```python
from build123d import *

# Parameters (mm, degrees)
BOSS_EXTRUDE1_DEPTH     = 200
SKETCH4_R               = 30
CUT_EXTRUDE1_DEPTH      = 60
SHELL1_T                = -20
BOSS_EXTRUDE2_DEPTH     = 200
SKETCH6_R               = 115
CUT_EXTRUDE3_DEPTH      = 50
CUT_EXTRUDE4_DEPTH      = 716.017482304
CUT_EXTRUDE4_DEPTH_BACK = 716.017482304
SKETCH7_R               = 30


with BuildPart() as part:
    # Sketch1 → Boss-Extrude1 (new body)
    with BuildSketch(Plane(origin=(0, 0, 0), x_dir=(1, 0, 0), z_dir=(0, 1, 0))):
        with BuildLine():
            Line((-220, 270), (220, 270))
            ThreePointArc((220, 270), (255.355339059, 255.355339059), (270, 220))
            Line((270, 220), (270, -220))
            ThreePointArc((270, -220), (255.355339059, -255.355339059), (220, -270))
            Line((220, -270), (-220, -270))
            ThreePointArc((-220, -270), (-255.355339059, -255.355339059), (-270, -220))
            Line((-270, -220), (-270, 220))
            ThreePointArc((-270, 220), (-255.355339059, 255.355339059), (-220, 270))
        make_face()
    extrude(amount=BOSS_EXTRUDE1_DEPTH)

    # Sketch4 → Cut-Extrude1 (cut)
    with BuildSketch(Plane(origin=(0, 200, 0), x_dir=(1, 0, 0), z_dir=(0, 1, 0))):
        with Locations(Location((0, 160, 0), (0, 0, 270))):
            Circle(SKETCH4_R)
        with Locations(Location((160, 0, 0), (0, 0, 270))):
            Circle(SKETCH4_R)
        with Locations(Location((0, -160, 0), (0, 0, 270))):
            Circle(SKETCH4_R)
        with Locations(Location((-160, 0, 0), (0, 0, 270))):
            Circle(SKETCH4_R)
    extrude(amount=-CUT_EXTRUDE1_DEPTH, mode=Mode.SUBTRACT)

    # Shell1
    shell1_openings = [part.faces().sort_by_distance(p)[0] for p in [
        (0, 0, 0),
    ]]
    offset(amount=SHELL1_T, openings=shell1_openings, kind=Kind.INTERSECTION)

    # Sketch5 → Boss-Extrude2 (add)
    with BuildSketch(Plane(origin=(0, 0, 0), x_dir=(1, 0, 0), z_dir=(0, 1, 0))):
        with BuildLine():
            Line((-255, 305), (255, 305))
            ThreePointArc((255, 305), (290.355339059, 290.355339059), (305, 255))
            Line((305, 255), (305, -255))
            ThreePointArc((305, -255), (290.355339059, -290.355339059), (255, -305))
            Line((255, -305), (-255, -305))
            ThreePointArc((-255, -305), (-290.355339059, -290.355339059), (-305, -255))
            Line((-305, -255), (-305, 255))
            ThreePointArc((-305, 255), (-290.355339059, 290.355339059), (-255, 305))
        make_face()
        with BuildLine():
            Line((-220, 270), (220, 270))
            ThreePointArc((220, 270), (255.355339059, 255.355339059), (270, 220))
            Line((270, 220), (270, -220))
            ThreePointArc((270, -220), (255.355339059, -255.355339059), (220, -270))
            Line((220, -270), (-220, -270))
            ThreePointArc((-220, -270), (-255.355339059, -255.355339059), (-270, -220))
            Line((-270, -220), (-270, 220))
            ThreePointArc((-270, 220), (-255.355339059, 255.355339059), (-220, 270))
        make_face(mode=Mode.SUBTRACT)
    extrude(amount=BOSS_EXTRUDE2_DEPTH)

    # Sketch6 → Cut-Extrude3 (cut)
    with BuildSketch(Plane(origin=(310, 0, 0), x_dir=(0, 0, -1), z_dir=(1, 0, 0))):
        with Locations((0, 61.568690233)):
            Circle(SKETCH6_R)
    cut_extrude3 = extrude(amount=-CUT_EXTRUDE3_DEPTH, mode=Mode.SUBTRACT)

    # Sketch7 → Cut-Extrude4 (cut, two sides: drawn at the far end of the back side and taken through both)
    with BuildSketch(Plane(origin=(310, 0, 0), x_dir=(0, 0, -1), z_dir=(1, 0, 0)).offset(-CUT_EXTRUDE4_DEPTH_BACK)):
        with Locations((0, 61.568690233)):
            Circle(SKETCH7_R)
    extrude(amount=CUT_EXTRUDE4_DEPTH + CUT_EXTRUDE4_DEPTH_BACK, mode=Mode.SUBTRACT)

    # Mirror1: Cut-Extrude3 across plane
    add(cut_extrude3.mirror(Plane(origin=(0, 0, 0), x_dir=(0, 0, 1), z_dir=(1, 0, 0))), mode=Mode.SUBTRACT)


solid = part.part
```
Could you check a few things on this model? Use its own coordinates, in mm. A direction names the side the tool comes from. Round coordinates to 2 decimals unless told otherwise and drop trailing zeros. Loops run counter-clockwise (first coordinate to the right, second up) from the corner with the lowest first, then second, coordinate; pieces in that order, holes last. Notation, with made-up numbers: (57.5, 82) - (75.5, 82) arc R28 cw to (75.5, 117) - close; hole circle Ø1 at (4.5, 67). An arc over 180 degrees is marked (long way). Answer in a Markdown table with one row per item. Add a question column.
(1) If we section it at C-C (z = -160): Please give me the cut outline in (x, y), plus the area to 3 significant figures.
(2) I'm going to push flat-ended pins straight in: pin 1 (12 mm diameter, centred on x = 131, z = 34, fed in from -Y); pin 2 (5 mm diameter, centred on x = -209, z = 22, fed in from -Y); pin 3 (4 mm diameter, centred on y = 73, z = 90, fed in from -X). Where does each tip first touch, or does it pass through?
(3) If we mould it in two halves opening along Z, with no side actions, what happens to faces 1 (the face through (-240.979, 88.74, 241.445)), 2 (the face through (-4, 99, -305)), 3 (the face through (4, 200, -4)), 4 (the face through (-250, 109, 3))? For each: pulls with the +Z half, pulls with the -Z half, needs draft (parallel to the pull), parting line crosses it, or undercut.
(4) If we section it at A-A (x = 0): Please give me the cut outline in (y, z).
(5) If we section it at B-B (y = 22): Please give me the cut outline in (x, z), plus the area to 3 significant figures.
(6) I need wall thicknesses on line 1 along X through (y, z) = (173, -160); line 2 along X through (y, z) = (172.5, 0); line 3 along X through (y, z) = (23, -6.5). Which ranges of each line are inside material? Lowest first, please.
(7) For faces 5 (the face through (-44, 0, -273)), 6 (the face through (260, 90, -24)), 7 (the face through (-159, 120, -1)), 8 (the face through (-282.815, 176.517, -3.438)), 9 (the face through (1.32, 170.42, 130.03)), which set-ups out of +Z, -Z, +X, -X, +Y, -Y let a thin tool reach every point of the face, with its end or its side?
Model answer:
| question | item | result |
|---|---|---|
| 1 | outline | (-305, 0) - (-250, 0) - (-250, 180) - (-50, 180) - (-50, 120) - (50, 120) - (50, 180) - (250, 180) - (250, 0) - (305, 0) - (305, 200) - (30, 200) - (30, 140) - (-30, 140) - (-30, 200) - (-305, 200) - close |
| 1 | area | 34,400 mm² |
| 2 | pin 1 | stops at y = 120 |
| 2 | pin 2 | stops at y = 180 |
| 2 | pin 3 | stops at x = -260 |
| 3 | face 1 | undercut |
| 3 | face 2 | pulls with the -Z half |
| 3 | face 3 | needs draft |
| 3 | face 4 | undercut |
| 4 | outline | (0, -305) - (200, -305) - (200, -190) - (140, -190) - (140, -130) - (200, -130) - (200, 130) - (140, 130) - (140, 190) - (200, 190) - (200, 305) - (0, 305) - (0, 250) - (180, 250) - (180, 210) - (120, 210) - (120, 110) - (180, 110) - (180, -110) - (120, -110) - (120, -210) - (180, -210) - (180, -250) - (0, -250) - close |
| 5 | outline | (-305, -255) arc R50 ccw to (-255, -305) - (255, -305) arc R50 ccw to (305, -255) - (305, -107.98) - (260, -107.98) - (260, 107.98) - (305, 107.98) - (305, 255) arc R50 ccw to (255, 305) - (-255, 305) arc R50 ccw to (-305, 255) - (-305, 107.98) - (-260, 107.98) - (-260, -107.98) - (-305, -107.98) - close; hole (-250, -220) arc R30 ccw to (-220, -250) - (220, -250) arc R30 ccw to (250, -220) - (250, 220) arc R30 ccw to (220, 250) - (-220, 250) arc R30 ccw to (-250, 220) - close |
| 5 | area | 101,000 mm² |
| 6 | line 1 | x = -305 to -250, -50 to -30, 30 to 50, 250 to 305 |
| 6 | line 2 | x = -260 to -250, -210 to -190, -130 to -110, 110 to 130, 190 to 210, 250 to 260 |
| 6 | line 3 | x = -260 to -250, 250 to 260 |
| 7 | face 5 | +Z, -Z, +X, -X, -Y |
| 7 | face 6 | +X |
| 7 | face 7 | -Y |
| 7 | face 8 | -X |
| 7 | face 9 | +Y |
